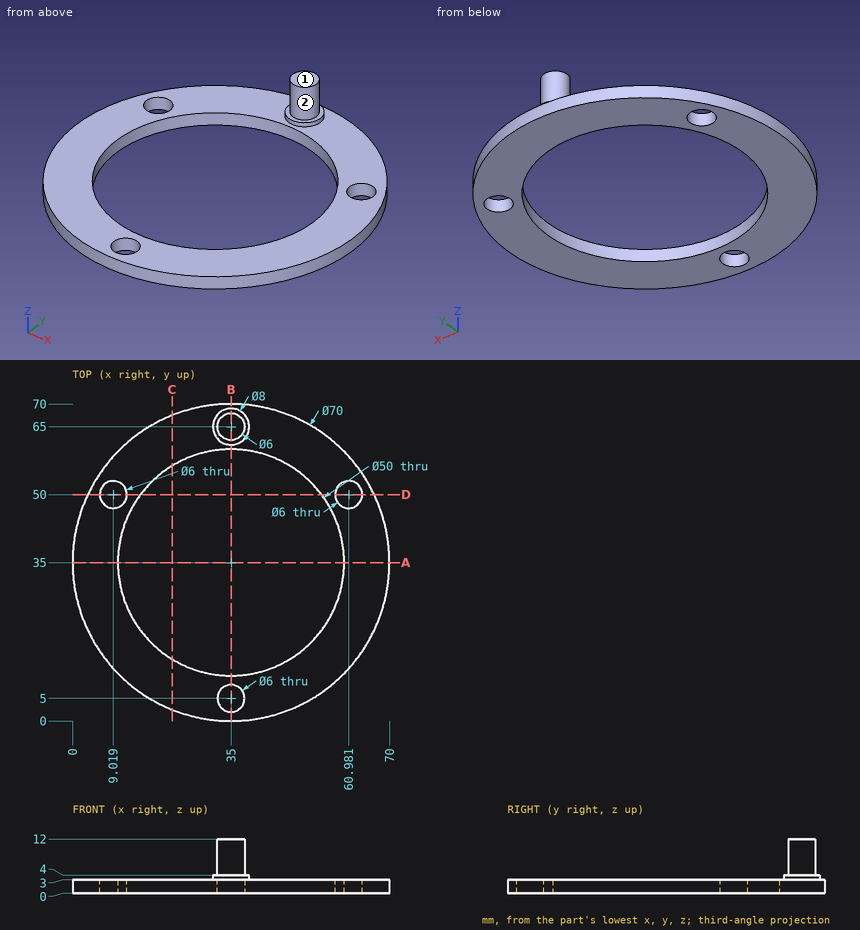
Check sheet for the drawn part. Datum: minimum x, y, z corner. Units: mm. A direction names the side the tool comes from. Round coordinates to 2 decimals unless told otherwise and drop trailing zeros. Loops run counter-clockwise (first coordinate to the right, second up) from the corner with the lowest first, then second, coordinate; pieces in that order, holes last. Notation, with made-up numbers: (-26, 52) - (26, 52) arc R16 ccw to (26, 72) - close; hole circle Ø11 at (4, 49.5). An arc over 180 degrees is marked (long way). Write each question's results on one line, items separated by ' | '. Start each with the question number.
Q1. Cross-section at B-B on x = 35. Enter the section's corners in (y, z).
Q2. Thickness scan on line 1 (Y direction, x = 35, z = 1); line 2 (Z direction, x = 16.5, y = 12); line 3 (Y direction, x = 35, z = 10). Record the ranges inside material, lowest first. Write a range as [from, to].
Q3. Cross-section at D-D on y = 50. Enter the section's corners in (x, z).
Q4. Gauge pin test, flat ends, axial feed: P1, Ø8, axis at x = 60.98, y = 50, coming from the +Z side; P2, Ø4, axis at x = 39, z = 4.5, coming from the +Y side; P3, Ø3.5, axis at x = 35, y = 5, coming from the -Z side; P4, Ø5, axis at x = 12, z = 2, coming from the +Y side. Record the tip position at first contact, or that the pin passes through.
Q5. Cross-section at C-C on x = 22. Enter the section's corners in (y, z).
Q6. Cross-section at A-A on y = 35. Enter the section's corners in (x, z).
Q7. Access from +Z, -Z, +X, -X, +Y, -Y to the whole of each face (thin tool, end or side, straight path). Record for the marked faces 1 and 2.
Answers below:
1) outline: (0, 0) - (2, 0) - (2, 3) - (0, 3) - close; (8, 0) - (10, 0) - (10, 3) - (8, 3) - close; (60, 0) - (70, 0) - (70, 3) - (69, 3) - (69, 4) - (68, 4) - (68, 12) - (62, 12) - (62, 4) - (61, 4) - (61, 3) - (60, 3) - close
2) line 1: y = [0, 2], [8, 10], [60, 70] | line 2: z = [0, 3] | line 3: y = [62, 68]
3) outline: (3.38, 0) - (6.02, 0) - (6.02, 3) - (3.38, 3) - close; (12.02, 0) - (15, 0) - (15, 3) - (12.02, 3) - close; (55, 0) - (57.98, 0) - (57.98, 3) - (55, 3) - close; (63.98, 0) - (66.62, 0) - (66.62, 3) - (63.98, 3) - close
4) P1: stops at z = 3 | P2: stops at y = 69.9 | P3: passes through | P4: stops at y = 63.37
5) outline: (2.5, 0) - (13.65, 0) - (13.65, 3) - (2.5, 3) - close; (56.35, 0) - (67.5, 0) - (67.5, 3) - (56.35, 3) - close
6) outline: (0, 0) - (10, 0) - (10, 3) - (0, 3) - close; (60, 0) - (70, 0) - (70, 3) - (60, 3) - close
7) face 1: +Z, +X, -X, +Y, -Y | face 2: +Z
